from build123d import *

# Parameters (mm, degrees)
F0_W     = 22.5
F0_H     = 37
F1_DEPTH = 18.8
F2_R     = 5
F4_D     = 3.3
F6_D     = 7.2


with BuildPart() as f1:
    # F0 (on Top) → F1 (new body)
    with BuildSketch(Plane.XY):
        Rectangle(F0_W, F0_H)
    extrude(amount=F1_DEPTH)

    # F2
    f2_edges = [f1.edges().sort_by_distance(p)[0] for p in [
        (11.25, 18.5, 9.4),
        (-11.25, 18.5, 9.4),
    ]]
    fillet(f2_edges, radius=F2_R)

    # F4 (through all)
    with Locations(Plane.XY.offset(18.8)):
        with Locations((-8.75, -13.3), (8.75, -13.3)):
            Hole(F4_D / 2)

    # F6 (through all)
    with Locations(Plane.XY.offset(18.8)):
        with Locations((0, 7.3)):
            Hole(F6_D / 2)


solid = f1.part
CAD build for the part. Positions are in the model's coordinates, mm. Coordinates: 2 decimals unless noted, no trailing zeros. Loops run counter-clockwise (first coordinate to the right, second up) from the corner with the lowest first, then second, coordinate; pieces in that order, holes last. Notation, with made-up numbers: (59, 61.5) - (113, 61.5) arc R19 cw to (113, 94.5) - close; hole circle Ø7 at (-18, 13.25). An arc over 180 degrees is marked (long way). Use one line per item in the form item = value. Start each with the question number.
1) Band-saw the part on D-D (x = 8.75). Give the cut face in (y, z).
2) Band-saw the part on B-B (y = -13.3). Give the cut face in (x, z), and give its area (3 significant figures).
3) Band-saw the part on A-A (x = 0). Give the cut face in (y, z).
4) Drill centre lines: L1, parallel to Y at x = 0, z = 4.5; L2, parallel to Y at x = 2.25, z = 4; L3, parallel to X at y = 10, z = 5.5. Where is each one in solid material? Low to high. Write a range as from..to.
5) Band-saw the part on C-C (z = 7.5). Give the cut face in (x, y), and give its area (3 significant figures).
6) Two-plate mould, pull along Y, no slides. Class faces 1 (the face through (-7.44, -14.3, 9.27)), 2 (the face through (0, -18.5, 9)), 3 (the face through (0.47, 10.87, 9.27)), 4 (the face through (-11.25, -3, 9)): +Y half, -Y half, draft (parallel to the pull), parting line (faces both ways), or undercut.
Check values:
q1.outline = (-18.5, 0) - (-14.95, 0) - (-14.95, 18.8) - (-18.5, 18.8) - close; (-11.65, 0) - (17.83, 0) - (17.83, 18.8) - (-11.65, 18.8) - close
q2.outline = (-11.25, 0) - (-10.4, 0) - (-10.4, 18.8) - (-11.25, 18.8) - close; (-7.1, 0) - (7.1, 0) - (7.1, 18.8) - (-7.1, 18.8) - close; (10.4, 0) - (11.25, 0) - (11.25, 18.8) - (10.4, 18.8) - close
q2.area = 299 mm2
q3.outline = (-18.5, 0) - (3.7, 0) - (3.7, 18.8) - (-18.5, 18.8) - close; (10.9, 0) - (18.5, 0) - (18.5, 18.8) - (10.9, 18.8) - close
q4.L1 = -18.5..3.7, 10.9..18.5
q4.L2 = -18.5..4.49, 10.11..18.5
q4.L3 = -11.25..-2.38, 2.38..11.25
q5.outline = (-11.25, -18.5) - (11.25, -18.5) - (11.25, 13.5) arc R5 ccw to (6.25, 18.5) - (-6.25, 18.5) arc R5 ccw to (-11.25, 13.5) - close; hole circle Ø3.3 at (-8.75, -13.3); hole circle Ø7.2 at (0, 7.3); hole circle Ø3.3 at (8.75, -13.3)
q5.area = 764 mm2
q6.face_1 = undercut
q6.face_2 = -Y half
q6.face_3 = undercut
q6.face_4 = draft
